```python
from build123d import *

# Parameters (mm, degrees)
CROQUIS1_R              = 2.6
CROQUIS1_R_2            = 1.5
CROQUIS1_W              = 12
CROQUIS1_H              = 4
SALIENTE_EXTRUIR1_DEPTH = 4.15
CROQUIS2_R              = 1.5
CORTAR_EXTRUIR1_DEPTH   = 10
REDONDEO2_R             = 2


with BuildPart() as part:
    # Croquis1 → Saliente-Extruir1 (new, symmetric)
    # profile 1 of 2: a face of its own
    with BuildSketch(Plane.XY):
        with BuildLine():
            Line((-14.490607503, -1040.48), (-14.490607503, -1037.604369418))
            Line((-14.490607503, -1037.604369418), (-14.490607503, -972.48))
            Line((-14.490607503, -972.48), (-22.490607503, -972.48))
            Line((-22.490607503, -972.48), (-22.490607503, -993.48))
            Line((-22.490607503, -993.48), (-22.490607503, -997.48))
            Line((-22.490607503, -997.48), (-22.490607503, -1024.48))
            Line((-22.490607503, -1024.48), (-22.490607503, -1040.48))
            ThreePointArc((-22.490607503, -1040.48), (-18.490607503, -1044.48), (-14.490607503, -1040.48))
        make_face()
        with Locations(Location((-18.490607503, -1040.48, 0), (0, 0, 180))):
            Circle(CROQUIS1_R, mode=Mode.SUBTRACT)
        with Locations(Location((-18.490607503, -1032.48, 0), (0, 0, 180))):
            Circle(CROQUIS1_R, mode=Mode.SUBTRACT)
        with Locations(Location((-18.490607503, -1024.48, 0), (0, 0, 180))):
            Circle(CROQUIS1_R, mode=Mode.SUBTRACT)
        with Locations(Location((-18.490607503, -987.48, 0), (0, 0, 180))):
            Circle(CROQUIS1_R_2, mode=Mode.SUBTRACT)
        with Locations(Location((-18.490607503, -977.48, 0), (0, 0, 180))):
            Circle(CROQUIS1_R_2, mode=Mode.SUBTRACT)
    # profile 2 of 2: a face of its own
    with BuildSketch(Plane.XY):
        with Locations((-28.490607503, -995.48)):
            Rectangle(CROQUIS1_W, CROQUIS1_H)
    extrude(amount=SALIENTE_EXTRUIR1_DEPTH, both=True)

    # Croquis2 → Cortar-Extruir1 (cut)
    with BuildSketch(Plane(origin=(0, -993.48, 0), x_dir=(1, 0, 0), z_dir=(0, 1, 0))):
        with Locations(Location((-30.490607503, 0, 0), (0, 0, 270))):
            Circle(CROQUIS2_R)
    extrude(amount=-CORTAR_EXTRUIR1_DEPTH, mode=Mode.SUBTRACT)

    # Redondeo2
    redondeo2_edges = [part.edges().sort_by_distance(p)[0] for p in [
        (-22.490607503, -997.48, 0),
    ]]
    fillet(redondeo2_edges, radius=REDONDEO2_R)


solid = part.part
```
The model under review builds one solid part; all positions refer to its coordinate system, in mm. A direction names the side the tool comes from. Round coordinates to 2 decimals unless told otherwise and drop trailing zeros. Write each loop counter-clockwise with the first axis right and the second up, starting at its lowest first coordinate (ties: lowest second). Pieces come first, ordered by that corner, then holes. Notation, with made-up numbers: M 38,38.25 L 61,38.25 A28 ccw 61,65.25 Z; hole C 4,-20 d11. An arc over 180 degrees is marked long. Use CSV: the item, a comma, the result in double quotes. Start each with the question number.
(1) We need section D-D, the plane y = -1032.48. State the section outline as (x, z) points.
(2) For line 1 along X through (y, z) = (-987.48, 0); line 2 along Y through (x, z) = (-16.25, -3); line 3 along X through (y, z) = (-995.7, 0), list the stretches that pass through material, from the lowest coordinate up.
(3) The part is to be moulded in two halves that separate along X. For faces 1 (the face through (-28.6, -993.48, 0.1)), 2 (the face through (-23.09, -998.05, 0.06)), 3 (the face through (-18.58, -1044.48, 0.06)), 4 (the face through (-18.152, -1043.058, -0.058)), say which applies: +X half, -X half, draft (parallel to the pull), parting line (faces both ways), or undercut.
(4) We need section C-C, the plane z = 3. State the section outline as (x, y) points.
(5) We need section A-A, the plane y = -987.48. State the section outline as (x, z) points, then the cut area to 3 significant figures.
(6) We need section B-B, the plane z = 0. State the section outline as (x, y) points, then the cut area to 3 significant figures.
(7) Tool access review of faces 5 (the face through (-28, -997.48, 0)), 6 (the face through (-22.491, -983, 0)), 7 (the face through (-18.165, -976.016, -0.058)): name each direction out of +Z, -Z, +X, -X, +Y, -Y from which nothing blocks a thin tool from reaching the whole face with its end or side.
(8) Clearance check with flat-ended pins moving along their axes: P1, Ø1.5, axis at x = -29.5, z = 0.5, coming from the +Y side; P2, Ø2.5, axis at x = -31, z = -2, coming from the -Y side; P3, Ø4, axis at y = -1013.5, z = 0, coming from the -X side. State where each tip first meets the part, or that it passes through.
Findings:
1,outline,"M -22.49,-4.15 L -21.09,-4.15 L -21.09,4.15 L -22.49,4.15 Z; M -15.89,-4.15 L -14.49,-4.15 L -14.49,4.15 L -15.89,4.15 Z"
2,line 1,"-22.49 to -19.99, -16.99 to -14.49"
2,line 2,"-1043.79 to -1041.8, -1039.16 to -1033.8, -1031.16 to -1025.8, -1023.16 to -972.48"
2,line 3,"-34.49 to -31.99, -28.99 to -14.49"
3,face 1,"draft"
3,face 2,"-X half"
3,face 3,"parting line"
3,face 4,"undercut"
4,outline,"M -34.49,-997.48 L -24.49,-997.48 A2 cw -22.49,-999.48 L -22.49,-1040.48 A4 ccw -14.49,-1040.48 L -14.49,-972.48 L -22.49,-972.48 L -22.49,-993.48 L -34.49,-993.48 Z; hole C -18.49,-1040.48 d5.2; hole C -18.49,-1032.48 d5.2; hole C -18.49,-1024.48 d5.2; hole C -18.49,-987.48 d3; hole C -18.49,-977.48 d3"
5,outline,"M -22.49,-4.15 L -19.99,-4.15 L -19.99,4.15 L -22.49,4.15 Z; M -16.99,-4.15 L -14.49,-4.15 L -14.49,4.15 L -16.99,4.15 Z"
5,area,"41.5 mm^2"
6,outline,"M -34.49,-997.48 L -31.99,-997.48 L -31.99,-993.48 L -34.49,-993.48 Z; M -28.99,-997.48 L -24.49,-997.48 A2 cw -22.49,-999.48 L -22.49,-1040.48 A4 ccw -14.49,-1040.48 L -14.49,-972.48 L -22.49,-972.48 L -22.49,-993.48 L -28.99,-993.48 Z; hole C -18.49,-1040.48 d5.2; hole C -18.49,-1032.48 d5.2; hole C -18.49,-1024.48 d5.2; hole C -18.49,-987.48 d3; hole C -18.49,-977.48 d3"
6,area,"528 mm^2"
7,face 5,"+Z, -Z, -X, -Y"
7,face 6,"+Z, -Z, -X, +Y"
7,face 7,"+Z, -Z"
8,P1,"y = -993.48"
8,P2,"y = -997.48"
8,P3,"x = -22.49"
